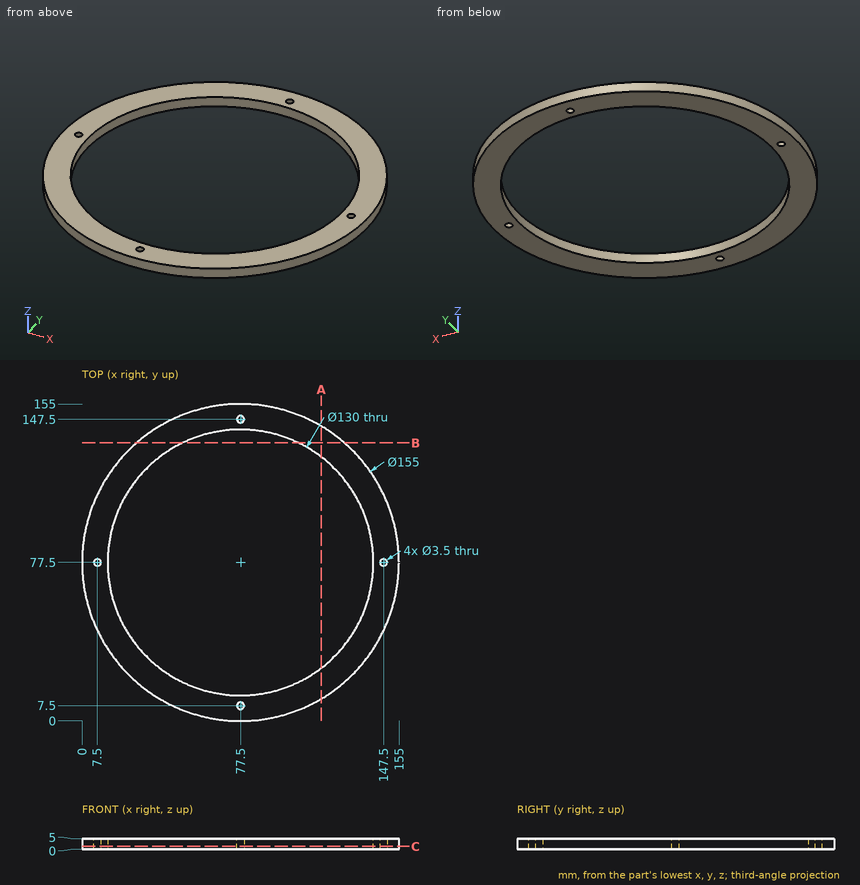
Geometry: see drawing. Coordinates: mm, zero at the bounding-box minimum. Round coordinates to 2 decimals unless told otherwise and drop trailing zeros. Loops run counter-clockwise (first coordinate to the right, second up) from the corner with the lowest first, then second, coordinate; pieces in that order, holes last. Notation, with made-up numbers: M 4,19 L 44,19 A20 ccw 44,36 Z; hole C 32.25,-14 d6. An arc over 180 degrees is marked long. Use a Markdown table: item, result. Add a question column.
1. Contact query for flat-ended pins moving along their axis: P1, Ø2, axis at x = 7.5, y = 77.5, coming from the +Z side; P2, Ø2, axis at x = 130.5, z = 1, coming from the +Y side; P3, Ø2, axis at x = 91.5, z = 1.5, coming from the -Y side; P4, Ø3, axis at x = 93, z = 2, coming from the +Y side (3 decimals). Output: stop coordinate, or through.
2. Line query: line 1 (Y direction, x = 77.5, z = 1.15); line 2 (X direction, y = 147.5, z = 1.25); line 3 (X direction, y = 105.5, z = 2.7). Output: solid intervals per line, ascending.
3. Section query A-A on x = 117. Return the cut outline in (y, z), then the cut area to 3 significant figures.
4. Section query C-C on z = 1.35. Return the cut outline in (x, y), then the cut area to 3 significant figures.
5. Section query B-B on y = 136. Return the cut outline in (x, z).
Reported:
| question | item | result |
|---|---|---|
| 1 | P1 | passes through |
| 1 | P2 | stops at y = 134.97 |
| 1 | P3 | stops at y = 1.1 |
| 1 | P4 | stops at y = 153.725 |
| 2 | line 1 | y = 0 to 5.75, 9.25 to 12.5, 142.5 to 145.75, 149.25 to 155 |
| 2 | line 2 | x = 44.24 to 75.75, 79.25 to 110.76 |
| 2 | line 3 | x = 5.23 to 18.84, 136.16 to 149.77 |
| 3 | outline | M 10.82,0 L 25.88,0 L 25.88,5 L 10.82,5 Z; M 129.12,0 L 144.18,0 L 144.18,5 L 129.12,5 Z |
| 3 | area | 151 mm² |
| 4 | outline | C 77.5,77.5 d155; hole C 7.5,77.5 d3.5; hole C 77.5,77.5 d130; hole C 77.5,7.5 d3.5; hole C 77.5,147.5 d3.5; hole C 147.5,77.5 d3.5 |
| 4 | area | 5,560 mm² |
| 5 | outline | M 26.67,0 L 49.17,0 L 49.17,5 L 26.67,5 Z; M 105.83,0 L 128.33,0 L 128.33,5 L 105.83,5 Z |
